The listing builds one solid part. Answer for the finished solid, in the listing's coordinates (mm). Face numbers are marked on the shaded views. Coordinates: 2 decimals unless noted, no trailing zeros. Order: outer loops, then holes, each group sorted by start corner. A loop starts at its lowest first (then second) coordinate and runs counter-clockwise, first axis right, second up. Notation, with made-up numbers: (-6, 40) -> (20, 40) arc R21 ccw to (20, 54) -> close; hole circle Ø7 at (73, 53.25). An arc over 180 degrees is marked (long way). Return JSON: item names as keys, results as strings.
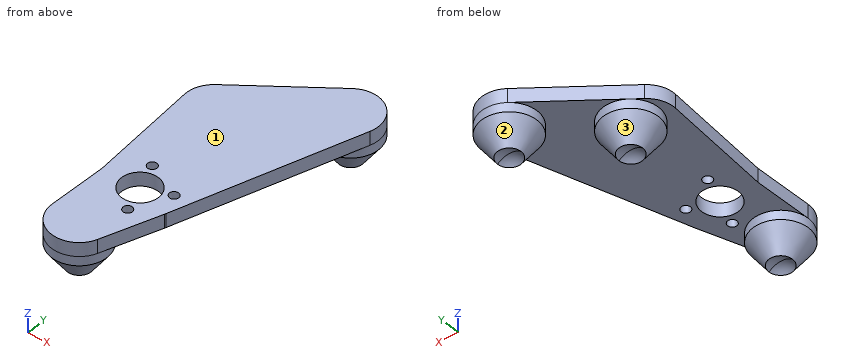
from build123d import *
from build123d.topology import SkipClean

# Parameters (mm, degrees)
BOSS_EXTRUDE1_DEPTH = 3
BOSS_EXTRUDE2_DEPTH = 3
SKETCH3_R           = 4
CUT_EXTRUDE1_DEPTH  = 50
SKETCH4_R           = 1
CUT_EXTRUDE2_DEPTH  = 10
BOSS_EXTRUDE3_START = -7
SKETCH1_4_R         = 6
BOSS_EXTRUDE3_DEPTH = 7
BOSS_EXTRUDE4_START = -7
SKETCH2_4_R         = 6
BOSS_EXTRUDE4_DEPTH = 7
CHAMFER1_SIZE       = 5
CHAMFER1_SIZE_2     = 3.501037691


with BuildPart() as part:
    # Sketch1 → Boss-Extrude1 (new body)
    with BuildSketch(Plane.XY):
        with BuildLine():
            ThreePointArc((-7.862783113, 28.36246747), (-9.674812704, 26.016588816), (-10.142674299, 23.089524856))
            Line((-10.142674299, 23.089524856), (-7.966824047, -0.727814955))
            ThreePointArc((-7.966824047, -0.727814955), (-0.830270862, -7.956798998), (7.644946217, -2.356861757))
            Line((7.644946217, -2.356861757), (19.414515396, 35.820058514))
            ThreePointArc((19.414515396, 35.820058514), (17.084366379, 42.528936958), (9.985578884, 42.314786229))
            Line((9.985578884, 42.314786229), (-7.862783113, 28.36246747))
        make_face()
    extrude(amount=BOSS_EXTRUDE1_DEPTH)

    # Sketch2 → Boss-Extrude2 (add)
    with BuildSketch(Plane.XY):
        with BuildLine():
            Line((-7.9983883, 0.16057583), (-8.256217535, -12.682068917))
            ThreePointArc((-8.256217535, -12.682068917), (-3.299315376, -18.711347307), (3.420783665, -14.741039282))
            Line((3.420783665, -14.741039282), (7.570946632, -2.584717991))
            ThreePointArc((7.570946632, -2.584717991), (-1.389185421, -7.878462024), (-7.9983883, 0.16057583))
        make_face()
    extrude(amount=BOSS_EXTRUDE2_DEPTH)

    # Sketch3 → Cut-Extrude1 (cut)
    with BuildSketch(Plane.XY.offset(3)):
        Circle(SKETCH3_R)
    extrude(amount=-CUT_EXTRUDE1_DEPTH, mode=Mode.SUBTRACT)

    # Sketch4 → Cut-Extrude2 (cut)
    with BuildSketch(Plane.XY.offset(3)):
        with Locations((2.135535698, -5.607092587)):
            Circle(SKETCH4_R)
        with Locations((-2.135535698, 5.607092587)):
            Circle(SKETCH4_R)
        with Locations((5.607092587, 2.135535698)):
            Circle(SKETCH4_R)
    extrude(amount=-CUT_EXTRUDE2_DEPTH, mode=Mode.SUBTRACT)

    # Sketch1<4> → Boss-Extrude3 (add)
    with SkipClean():  # the faces are left unmerged after this step: merging them gives an invalid solid
        with BuildSketch(Plane.XY.offset(BOSS_EXTRUDE3_START)):
            with Locations(Location((13.680805733, 37.587704831, 0), (0, 0, 128.01524628))):
                Circle(SKETCH1_4_R)
            with Locations((-2.167556264, 25.198814555)):
                Circle(SKETCH1_4_R)
        extrude(amount=BOSS_EXTRUDE3_DEPTH)

    # Sketch2<4> → Boss-Extrude4 (add)
    with SkipClean():  # the faces are left unmerged after this step: merging them gives an invalid solid
        with BuildSketch(Plane.XY.offset(BOSS_EXTRUDE4_START)):
            with Locations(Location((-2.25742631, -12.802500789, 0), (0, 0, 178.849883098))):
                Circle(SKETCH2_4_R)
        extrude(amount=BOSS_EXTRUDE4_DEPTH)

    # Sketch5 one side → Cut-Revolve1 (revolve, cut)
    with SkipClean():  # the faces are left unmerged after this step: merging them gives an invalid solid
        with BuildSketch(Plane(origin=(13.680805733, 0, 0), x_dir=(0, 0, -1), z_dir=(1, 0, 0))):
            with BuildLine():
                ThreePointArc((10, 33.587704831), (12.828427125, 34.759277707), (14, 37.587704831))
                ThreePointArc((14, 37.587704831), (12.828427125, 40.416131956), (10, 41.587704831))
                Line((10, 41.587704831), (10, 33.587704831))
            make_face()
        revolve(axis=Axis((13.680805733, 41.587704831, -10), (0, -1, 0)), mode=Mode.SUBTRACT)

    # Sketch6 → Cut-Revolve2 (revolve, cut)
    with SkipClean():  # the faces are left unmerged after this step: merging them gives an invalid solid
        with BuildSketch(Plane(origin=(-2.167556264, 0, 0), x_dir=(0, 0, -1), z_dir=(1, 0, 0))):
            with BuildLine():
                ThreePointArc((14, 25.198814555), (12.828427125, 28.02724168), (10, 29.198814555))
                Line((10, 29.198814555), (10, 21.198814555))
                ThreePointArc((10, 21.198814555), (12.828427125, 22.37038743), (14, 25.198814555))
            make_face()
            with BuildLine():
                Line((10, 21.198814555), (10, 29.198814555))
                ThreePointArc((10, 29.198814555), (6, 25.198814555), (10, 21.198814555))
            make_face()
        revolve(axis=Axis((-2.167556264, 29.198814555, -10), (0, -1, 0)), mode=Mode.SUBTRACT)

    # Sketch7 → Cut-Revolve3 (revolve, cut)
    with SkipClean():  # the faces are left unmerged after this step: merging them gives an invalid solid
        with BuildSketch(Plane(origin=(-2.25742631, 0, 0), x_dir=(0, 0, -1), z_dir=(1, 0, 0))):
            with BuildLine():
                ThreePointArc((14, -12.802500789), (12.828427125, -9.974073664), (10, -8.802500789))
                Line((10, -8.802500789), (10, -16.802500789))
                ThreePointArc((10, -16.802500789), (12.828427125, -15.630927914), (14, -12.802500789))
            make_face()
            with BuildLine():
                Line((10, -16.802500789), (10, -8.802500789))
                ThreePointArc((10, -8.802500789), (6, -12.802500789), (10, -16.802500789))
            make_face()
        revolve(axis=Axis((-2.25742631, -8.802500789, -10), (0, -1, 0)), mode=Mode.SUBTRACT)

    # Chamfer1
    # the kernel refuses this chamfer: 5, 3.501037691 mm, written as the material it takes off along each edge
    with BuildSketch(Plane(origin=(-2.25742631, -12.802500789, -7), x_dir=(-0.9997985375420249, 0.020071978697384193, 0), z_dir=(0.020071978697384193, 0.9997985375420249, 0))) as chamfer1_piece_1:
        Polygon((6, CHAMFER1_SIZE), (6 - CHAMFER1_SIZE_2, 0), (6, 0), align=None)
    revolve(axis=Axis((-2.25742631, -12.802500789, -7), (0, 0, 1)), mode=Mode.SUBTRACT)
    with BuildSketch(Plane(origin=(13.680805733, 37.587704831, -7), x_dir=(-0.615871141442135, 0.7878468995552129, 0), z_dir=(0.7878468995552129, 0.615871141442135, 0))) as chamfer1_piece_2:
        Polygon((6, CHAMFER1_SIZE), (6 - CHAMFER1_SIZE_2, 0), (6, 0), align=None)
    revolve(axis=Axis((13.680805733, 37.587704831, -7), (0, 0, 1)), mode=Mode.SUBTRACT)
    with BuildSketch(Plane(origin=(-2.167556264, 25.198814555, -7), x_dir=(1, 0, 0), z_dir=(0, -1, 0))) as chamfer1_piece_3:
        Polygon((6, CHAMFER1_SIZE), (6 - CHAMFER1_SIZE_2, 0), (6, 0), align=None)
    revolve(axis=Axis((-2.167556264, 25.198814555, -7), (0, 0, 1)), mode=Mode.SUBTRACT)


solid = part.part
1. Each of these flat-tipped pins is pushed along its axis until it touches: pin 1 Ø5 at (x, y) = (0, 0) entering from +Z; pin 2 Ø1.5 at (x, y) = (1, 28.5) entering from -Z; pin 3 Ø2.5 at (x, y) = (5.61, 2.14) entering from -Z; pin 4 Ø1.5 at (x, z) = (-4, -3.5) entering from -Y. Where does it stop, or does it pass through?
Answer block:
{"pin 1": "passes through", "pin 2": "stops at z = -5.11", "pin 3": "stops at z = 0", "pin 4": "stops at y = -18.04"}
2. Consider line 1 (Z direction, x = -8.25, y = 20.5); line 2 (Y direction, x = -4, z = -4.25); line 3 (Y direction, x = -4.25, z = -3). Determine where each line is inside the solid, lowest interval first. Write a range as from..to.
Answer block:
{"line 1": "z = 0..3", "line 2": "y = -16.87..-8.74, 21.17..29.23", "line 3": "y = -17.71..-7.89, 20.33..30.07"}
3. Determine the mould class of the marked faces 1, 2 and 3 for opening direction Y: pulls with the +Y half, pulls with the -Y half, needs draft (parallel to the pull), parting line crosses it, or undercut.
Answer block:
{"face 1": "needs draft", "face 2": "parting line crosses it", "face 3": "undercut"}
4. The part is cut by section C-C on z = -5. Give the vertices of the cut face in (x, y), and give its area (3 significant figures).
Answer block:
{"outline": "circle Ø7.8 at (-2.26, -12.8); circle Ø7.8 at (-2.17, 25.2); circle Ø7.8 at (13.68, 37.59)", "area": "143 mm2"}
5. The part is cut by section B-B on x = -2. Give the number of separate pieces and of enclosed holes in the cut face, and give its area (3 significant figures).
Answer block:
{"separate pieces": "3", "enclosed holes": "0", "area": "254 mm2"}
6. The part is cut by section A-A on z = -1. Give the vertices of the cut face in (x, y).
Answer block:
{"outline": "circle Ø12 at (-2.26, -12.8); circle Ø12 at (-2.17, 25.2); circle Ø12 at (13.68, 37.59)"}
